Can you work these out from the drawing? Everything is in mm from the part's minimum corner. Round coordinates to 2 decimals unless told otherwise and drop trailing zeros. Write each loop counter-clockwise with the first axis right and the second up, starting at its lowest first coordinate (ties: lowest second). Pieces come first, ordered by that corner, then holes. Notation, with made-up numbers: (20, 51.5) -> (60, 51.5) arc R21 cw to (60, 66.5) -> close; hole circle Ø5 at (17.25, -4). An arc over 180 degrees is marked (long way). Write item = value, one per line. Start each with the question number.
1) If I drill on line 1 (Y direction, x = 59, z = 2.4); line 2 (X direction, y = 19, z = 1.8); line 3 (Y direction, x = 44.5, z = 1.75) (1 decimal), over which ranges is the centre line in solid material (lowest first)?
2) Imagine slicing it at D-D, the plane x = 96.5. Please give me the cut outline in (y, z), then the cut area to 3 significant figures.
3) Imagine slicing it at A-A, the plane x = 60. Please give me the cut outline in (y, z).
4) Imagine slicing it at B-B, the plane y = 15. Please give me the cut outline in (x, z), then the cut area to 3 significant figures.
5) Imagine slicing it at C-C, the plane z = 3.3. Please give me the cut outline in (x, y) (1 decimal), then the cut area to 3 significant figures.
6) I'm going to push flat-ended pins straight in: pin 1 (1.5 mm diameter, centred on x = 50.5, z = 3, fed in from -Y); pin 2 (1.5 mm diameter, centred on y = 11, z = 2.5, fed in from +X); pin 3 (1 mm diameter, centred on y = 49, z = 3, fed in from +X); pin 4 (3 mm diameter, centred on x = 99.5, y = 81, fed in from -Z). Where does each tip first touch, or does it pass through?
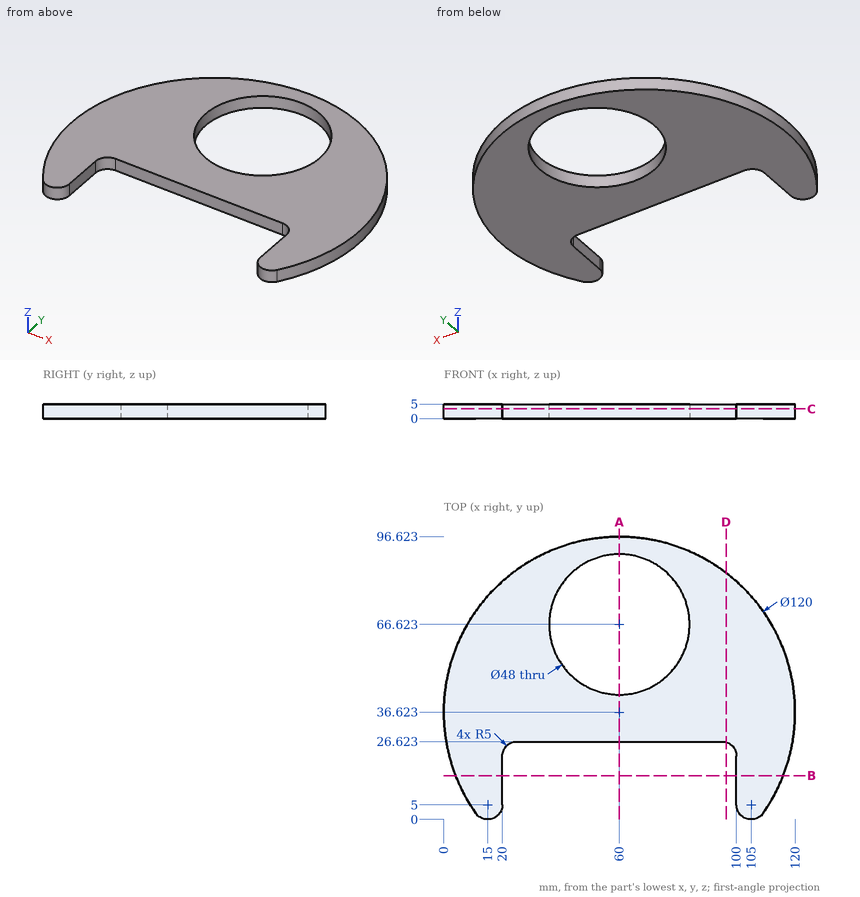
Reported:
q1.line_1 = 26.62 to 42.64, 90.6 to 96.61
q1.line_2 = 2.65 to 20, 100 to 117.35
q1.line_3 = 26.6 to 48.3, 84.9 to 94.6
q2.outline = (26.39, 0) -> (84.24, 0) -> (84.24, 5) -> (26.39, 5) -> close
q2.area = 289 mm²
q3.outline = (26.62, 0) -> (42.62, 0) -> (42.62, 5) -> (26.62, 5) -> close; (90.62, 0) -> (96.62, 0) -> (96.62, 5) -> (90.62, 5) -> close
q4.outline = (4.03, 0) -> (20, 0) -> (20, 5) -> (4.03, 5) -> close; (100, 0) -> (115.97, 0) -> (115.97, 5) -> (100, 5) -> close
q4.area = 160 mm²
q5.outline = (10.9, 2.1) arc R5 ccw to (20, 5) -> (20, 21.6) arc R5 cw to (25, 26.6) -> (95, 26.6) arc R5 cw to (100, 21.6) -> (100, 5) arc R5 ccw to (109.1, 2.1) arc R60 ccw (long way) to start; hole circle Ø48 at (60, 66.6)
q5.area = 5,820 mm²
q6.pin_1 = 26.62
q6.pin_2 = 114.6
q6.pin_3 = 118.81
q6.pin_4 = 0
